Autodesk Inventor part; units mm, degrees
ref_plane "WorkPlane1" through (0, 0, 0) normal (0, 0, 1) x (1, 0, 0)
ref_plane "MSC_PF1" through (0, 0, 0) normal (1, 0, 0) x (0, 1, 0)
ref_plane "MSC_PT1" through (0, 0, 0) normal (0, 0, -1) x (-1, 0, 0)
ref_plane "WorkPlane1" through (0, 0, 0) normal (0, 0, 1) x (1, 0, 0)
sketch "Skizze1" plane through (0, 0, 0) normal (0, 0, 1) x (1, 0, 0)
  point P0 (0, 0)
sketch "Skizze2" plane through (0, 0, 0) normal (0, 0, 1) x (1, 0, 0)
  line L0 (-9, 5.1963) -> (-9, -5.1963)
  line L1 (0, 10.3922) -> (-9, 5.1963)
  line L2 (9, 5.1963) -> (0, 10.3922)
  line L3 (9, -5.1963) -> (9, 5.1963)
  line L4 (0, -10.3922) -> (9, -5.1963)
  line L5 (-9, -5.1963) -> (0, -10.3922)
  circle A0 centre (0, 0) radius 9 construction
  dimension "d1" = 18
  dimension "d29" = 0
  dimension "d30" = 0
extrude "Extrusion1" add sketch "Skizze2" along normal blind 7.5
sketch "Skizze3" plane through (0, 0, 0) normal (1, 0, 0) x (0, 1, 0)
  line L0 (9, 7.5) -> (10.4922, 7.5)
  line L1 (10.4922, 6.6385) -> (9, 7.5)
  line L2 (10.4922, 7.5) -> (10.4922, 6.6385)
  line L3 (0, -1.5) -> (0, 9)
  line L4 (10.3922, 0) -> (10.3922, 7.5)
  dimension "d25" = 0.1
  dimension "d26" = 0
  dimension "d27" = 60
  dimension "d28" = 9
revolve "Drehung1" cut sketch "Skizze3" angle 360 about axis through (0, 0, -10) along (0, 0, 1)
sketch "Skizze4" plane through (0, 0, 0) normal (1, 0, 0) x (0, 1, 0)
  line L0 (0, -55) -> (0, 0)
  line L1 (-6, -55) -> (0, -55)
  line L2 (-6, 0) -> (-6, -55)
  line L3 (0, 0) -> (-6, 0)
  line L4 (0, -55) -> (0, 0)
  line L5 (-7.2, 0) -> (1.2, 0)
  line L6 (0, -66) -> (0, 11)
  dimension "d18" = 6
  dimension "d20" = 55
  dimension "d33" = 0
  dimension "d34" = 0
revolve "Drehung2" add sketch "Skizze4" angle 360 about axis through (0, 0, -55) along (0, 0, -1)
chamfer "Fase1" distance 0.875 angle 45 1 edges at (0, 6, -55)
fillet "Rundung1" radius 0.6 1 edges at (0, 6, 0)
thread "Gewinde1"
ref_plane "MSC_PF1" through (0, 0, 0) normal (1, 0, 0) x (0, 1, 0)
ref_plane "MSC_PT1" through (0, 0, 0) normal (0, 0, -1) x (-1, 0, 0)
equation "\"d22\" = 0.5 * PTC"
equation "\"d23\" = 0.5 * PTC"
equation "\"d1\" = ParS"
equation "\"d6\" = ParK"
equation "\"d24\" = r"
equation "\"d28\" = 0.5 * ParS"
equation "\"d18\" = 0.5 * NND"
equation "\"d20\" = NLG"
equation "\"NND\" = 12"
equation "\"NLG\" = 55"
equation "\"PTC\" = 1.75"
equation "\"ParK\" = 7.5"
equation "\"ParS\" = 18"
equation "\"msp_es\" = 0.577367 * ParS"
equation "\"r\" = 0.6"
equation "\"THREADDIA\" = NND"
equation "\"K1\" = 4.94"
properties part number "DIN EN ISO 4016 - M12x55" material "Stahl"
Geometry: final body of the model. Coordinates: model frame, mm. A direction names the side the tool comes from. Give positions to 0.01 mm unless a question says otherwise; leave off trailing zeros. Write each loop counter-clockwise with the first axis right and the second up, starting at its lowest first coordinate (ties: lowest second). Pieces come first, ordered by that corner, then holes. Notation, with made-up numbers: M 76.25,9.25 L 98.25,9.25 A28 ccw 98.25,44.25 Z; hole C 32,71.5 d3. An arc over 180 degrees is marked long. Answer in a Markdown table with one row per item. Add a question column.
(1) Section A-A on z = -12.5. Return loops of the section in (x, y), and give its area (3 significant figures).
(2) Reachability of faces 1 (the flat face through (0, -7, 0)), 2 (the flat face through (-4.44, 7.83, 3.7)) from +Z, -Z, +X, -X, +Y, -Y: full face, straight path, thin tool, end or side. Return the list, or none.
(3) First-contact query: pin 1 (5 mm diameter, centred on y = 5.5, z = -28, fed in from +X); pin 2 (1 mm diameter, centred on y = -3, z = -47, fed in from -X); pin 3 (5 mm diameter, centred on x = -1, z = -36.5, fed in from +Y). Flat tips, straight axial feed; report the tip coordinate or a pass-through.
(4) Ray query, line 1 (Z direction, x = 3.75, y = -5.5); line 2 (Y direction, x = -0.25, z = -47). Return the intervals inside material, ascending.
Result set:
| question | item | result |
|---|---|---|
| 1 | outline | C 0,0 d12 |
| 1 | area | 113 mm^2 |
| 2 | face 1 | -Z |
| 2 | face 2 | +Z, -Z, -X, +Y |
| 3 | pin 1 | stops at x = 5.2 |
| 3 | pin 2 | stops at x = -5.45 |
| 3 | pin 3 | stops at y = 6 |
| 4 | line 1 | z = 0 to 7.5 |
| 4 | line 2 | y = -5.99 to 5.99 |
